For this review, take the finished solid that the model builds, in its own axes (mm). Coordinates: 2 decimals unless noted, no trailing zeros. Loops run counter-clockwise (first coordinate to the right, second up) from the corner with the lowest first, then second, coordinate; pieces in that order, holes last. Notation, with made-up numbers: M 78.25,88 L 125.25,88 A32 cw 125.25,114 Z; hole C -15,88.25 d10. An arc over 180 degrees is marked long. Put each result on its own line as item: value.
```python
from build123d import *

# Parameters (mm, degrees)
SKETCH_W     = 125
SKETCH_H     = 125
SKETCH_R     = 52.5
PAD_DEPTH    = 35
SKETCH001_W  = 131.958801
SKETCH001_H  = 149.735626
POCKET_DEPTH = 35.001


with BuildPart() as part:
    # Sketch → Pad (new body)
    with BuildSketch(Plane.XY):
        Rectangle(SKETCH_W, SKETCH_H)
        Circle(SKETCH_R, mode=Mode.SUBTRACT)
    extrude(amount=PAD_DEPTH)

    # Sketch001 → Pocket (cut, through all)
    with BuildSketch(Plane.XY):
        with Locations((65.9794, -4.983963)):
            Rectangle(SKETCH001_W, SKETCH001_H)
    extrude(amount=POCKET_DEPTH, mode=Mode.SUBTRACT)


solid = part.part
```
(1) Add section D-D (y = 0). Write out the cut boundary in (x, z), plus the area to 3 significant figures.
Determined:
outline: M -62.5,0 L -52.5,0 L -52.5,35 L -62.5,35 Z
area: 350 mm^2
(2) Add section B-B (z = 26). Write out the cut boundary in (x, y).
Determined:
outline: M -62.5,-62.5 L 0,-62.5 L 0,-52.5 A52.5 cw 0,52.5 L 0,62.5 L -62.5,62.5 Z
(3) Add section A-A (x = -10). Write out the cut boundary in (y, z).
Determined:
outline: M -62.5,0 L -51.54,0 L -51.54,35 L -62.5,35 Z; M 51.54,0 L 62.5,0 L 62.5,35 L 51.54,35 Z
(4) Draft analysis for pull direction Y (two halves, no side actions). For faces 1 (the flat face through (-53, 1, 35)), 2 (the flat face through (-32, 62.5, 17)), 3 (the cylindrical face through (-52.487, 1.154, 17.255)), 4 (the flat face through (-32, -62.5, 17)), state which applies: +Y half, -Y half, draft (parallel to the pull), parting line (faces both ways), or undercut.
Determined:
face 1: draft
face 2: +Y half
face 3: undercut
face 4: -Y half
(5) Add section C-C (x = -47). Write out the cut boundary in (y, z), plus the area to 3 significant figures.
Determined:
outline: M -62.5,0 L -23.39,0 L -23.39,35 L -62.5,35 Z; M 23.39,0 L 62.5,0 L 62.5,35 L 23.39,35 Z
area: 2,740 mm^2
(6) For pin 1 (12 mm diameter, centred on y = -25, z = 20, fed in from +X); pin 2 (10 mm diameter, centred on y = -25, z = 4.5, fed in from +X); pin 3 (6 mm diameter, centred on y = 45.5, z = 16.5, fed in from +X); pin 4 (10 mm diameter, centred on x = -34.5, y = 45, fed in from -Z), all flat-tipped, find the tip position at first contact; note any pin that passes through.
Determined:
pin 1: stops at x = -42.37
pin 2: stops at x = -43.08
pin 3: stops at x = -20.1
pin 4: stops at z = 0
(7) Wall thickness on line 1 along Y through (x, z) = (-20.5, 21.5); line 2 along Y through (x, z) = (-10, 8.5); line 3 along X through (y, z) = (-30, 19.5): over which ranges is each line inside the solid? List them lowest first. Write a range as [from, to].
Determined:
line 1: y = [-62.5, -48.33], [48.33, 62.5]
line 2: y = [-62.5, -51.54], [51.54, 62.5]
line 3: x = [-62.5, -43.08]
